Verification items for the finished model (mm, model axes). A direction names the side the tool comes from. Give positions to 0.01 mm unless a question says otherwise; leave off trailing zeros. Loops run counter-clockwise (first coordinate to the right, second up) from the corner with the lowest first, then second, coordinate; pieces in that order, holes last. Notation, with made-up numbers: (17, -14) - (55, -14) arc R16 cw to (55, 0) - close; hole circle Ø4 at (24.5, -20). An arc over 180 degrees is marked (long way). One line per question, with ' | ' between items. Start each with the question number.
1. Depth check by flat-ended pin: pin 1 Ø8 at (y, z) = (-5, 11) entering from +X; pin 2 Ø1 at (y, z) = (1, 7) entering from -X; pin 3 Ø1.5 at (y, z) = (5, 13) entering from +X. Enter the tip coordinate at first touch or a pass-through.
2. Tool access check on faces 1 (the face through (-5.158, -3.955, 14.051)), 2 (the face through (0, 0, 0)), 3 (the face through (0, 7, 9)). Record the directions out of +Z, -Z, +X, -X, +Y, -Y that give a thin tool (end or side, any length) a straight path to the whole face; none if there is none.
3. Section check C-C, the plane x = -6. Enter the section's corners in (y, z).
4. Section check A-A, the plane y = 0. Enter the section's corners in (x, z).
5. Mould release check, pull along X, two halves, no side actions. Record for faces 4 (the face through (4.896, -2.03, 9.285)), 5 (the face through (0, 0, 1.2)), 6 (the face through (-5.158, -3.955, 4.437)), 7 (the face through (0, 7, 10.6)): +X half, -X half, draft (parallel to the pull), parting line (faces both ways), or undercut.
6. Section check B-B, the plane z = 6. Enter the section's corners in (x, y), then the cut area to 3 significant figures.
7. Thickness scan on line 1 along Y through (x, z) = (0, 11.75); line 2 along Z through (x, y) = (-1.5, -1.25); line 3 along Y through (x, z) = (-2.5, 2.5). Record the ranges inside material, lowest first. Write a range as from..to.
from build123d import *

# Parameters (mm, degrees)
F0_R     = 6.5
F1_DEPTH = 9
F2_R     = 8
F3_DEPTH = 1.6
F4_R     = 6.5
F5_DEPTH = 7
F6_T     = 1.2


# Not quite as in the source:
# - a shell that OpenCascade refuses in one call is made with other operations: the cavity is built on its own and cut out


with BuildPart() as f1:
    # F0 (on Top) → F1 (new body)
    with BuildSketch(Plane.XY):
        Circle(F0_R)
    extrude(amount=F1_DEPTH)

    # F2 (on face) → F3 (join)
    with BuildSketch(Plane.XY.offset(9)):
        Circle(F2_R)
    extrude(amount=F3_DEPTH)

    # F4 (on face) → F5 (join)
    with BuildSketch(Plane.XY.offset(10.6)):
        Circle(F4_R)
    extrude(amount=F5_DEPTH)

    # F6: shell of thickness 1.2, made by hand


with BuildPart() as f6_core1:
    # F6_t2: copy of F1
    add(f1.part)

    # the walls: a layer under each face that stays
    f6_faces = [f6_core1.faces().sort_by_distance(p)[0] for p in [
        (-8, 0, 9.8),
        (-5.3333333333, -5.3333333333, 9),
        (-5.3333333333, -5.3333333333, 10.6),
        (-6.5, 0, 4.5),
        (-6.5, 0, 14.1),
        (0, 0, 0),
    ]]
    thicken(f6_faces, amount=-F6_T, mode=Mode.SUBTRACT)

    # F6_s3 → F6_t4 (revolve, cut)
    with BuildSketch(Plane.XZ):
        Polygon((6.512, 8.988), (6.5, 10.2), (5.3, 10.2), (5.3, 9), align=None)
    revolve(axis=Axis((0, 0, 9), (0, 0, 1)), mode=Mode.SUBTRACT)

    # F6_s5 → F6_t6 (revolve, cut)
    with BuildSketch(Plane.XZ):
        Polygon((6.512, 10.612), (6.5, 9.4), (5.3, 9.4), (5.3, 10.6), align=None)
    revolve(axis=Axis((0, 0, 10.6), (0, 0, 1)), mode=Mode.SUBTRACT)


with BuildPart() as f1_1:
    add(f1.part)

    # what is left inside the walls is the cavity
    f6_cavity = [f6_core1.part.solids().sort_by_distance(p)[0] for p in [
        (-5.288, 0, 12.133333),
    ]]
    add(f6_cavity, mode=Mode.SUBTRACT)


solid = f1_1.part
Results list:
1) pin 1: x = 7.93 | pin 2: x = -6.48 | pin 3: x = 4.92
2) face 1: +Z | face 2: -Z, +X, -X, +Y, -Y | face 3: -Z
3) outline: (-5.29, 9) - (-2.5, 9) - (-2.5, 0) - (2.5, 0) - (2.5, 9) - (5.29, 9) - (5.29, 10.6) - (2.5, 10.6) - (2.5, 17.6) - (-2.5, 17.6) - (-2.5, 10.6) - (-5.29, 10.6) - close
4) outline: (-8, 9) - (-6.5, 9) - (-6.5, 0) - (6.5, 0) - (6.5, 9) - (8, 9) - (8, 10.6) - (6.5, 10.6) - (6.5, 17.6) - (5.3, 17.6) - (5.3, 1.2) - (-5.3, 1.2) - (-5.3, 17.6) - (-6.5, 17.6) - (-6.5, 10.6) - (-8, 10.6) - close
5) face 4: undercut | face 5: undercut | face 6: parting line | face 7: draft
6) outline: circle Ø13 at (0, 0); hole circle Ø10.6 at (0, 0) | area: 44.5 mm²
7) line 1: -6.5..-5.3, 5.3..6.5 | line 2: 0..1.2 | line 3: -6..-4.67, 4.67..6
